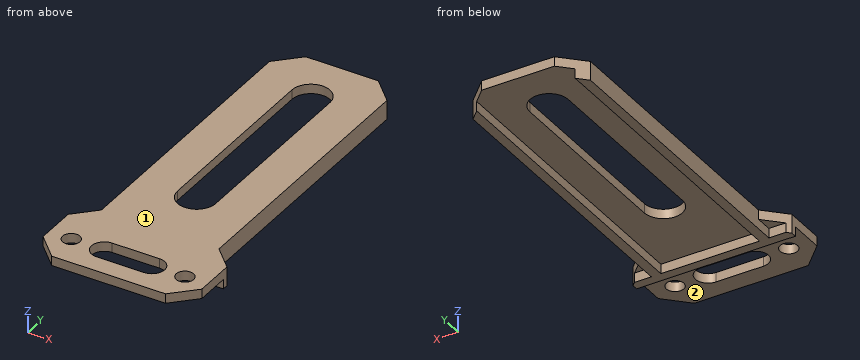
```python
from build123d import *

# Parameters (mm, degrees)
SKETCH1_R           = 2.75
BOSS_EXTRUDE1_DEPTH = 3
BOSS_EXTRUDE2_DEPTH = 3


with BuildPart() as part:
    # Sketch1 → Boss-Extrude1 (new body)
    with BuildSketch(Plane.XY):
        Polygon((7.071067812, 0), (42.928932188, 0), (50, 7.071067812), (50, 20), (43.5, 26.5), (43.5, 112.928932188), (36.428932188, 120), (13.571067812, 120), (6.5, 112.928932188), (6.5, 26.5), (0, 20), (0, 7.071067812), align=None)
        with Locations((7.1, 10)):
            Circle(SKETCH1_R, mode=Mode.SUBTRACT)
        with Locations(Location((42.9, 10, 0), (0, 0, 180))):
            Circle(SKETCH1_R, mode=Mode.SUBTRACT)
        with BuildLine():
            Line((19, 45.27), (19, 104))
            ThreePointArc((19, 104), (25, 110), (31, 104))
            Line((31, 104), (31, 45.27))
            ThreePointArc((31, 45.27), (25, 39.27), (19, 45.27))
        make_face(mode=Mode.SUBTRACT)
        with BuildLine():
            Line((17.5, 14), (32.5, 14))
            ThreePointArc((32.5, 14), (36.5, 10), (32.5, 6))
            Line((32.5, 6), (17.5, 6))
            ThreePointArc((17.5, 6), (13.5, 10), (17.5, 14))
        make_face(mode=Mode.SUBTRACT)
    extrude(amount=BOSS_EXTRUDE1_DEPTH)

    # Sketch2 → Boss-Extrude2 (add)
    with BuildSketch(Plane(origin=(0, 0, 0), x_dir=(-1, 0, 0), z_dir=(0, 0, -1))):
        Polygon((-50, 18.19), (0, 18.19), (0, 20), (-1.19, 21.19), (-6.5, 21.19), (-6.5, 112.928932188), (-9.5, 115.928932188), (-9.5, 21.19), (-40.5, 21.19), (-40.5, 115.928932188), (-43.5, 112.928932188), (-43.5, 21.19), (-48.81, 21.19), (-50, 20), align=None)
    extrude(amount=BOSS_EXTRUDE2_DEPTH)


solid = part.part
```
Input: part model. Units: mm. Frame: model coordinates. Face numbers are marked on the shaded views. Give positions to 0.01 mm unless a question says otherwise; leave off trailing zeros. Order: outer loops, then holes, each group sorted by start corner. A loop starts at its lowest first (then second) coordinate and runs counter-clockwise, first axis right, second up.
1. Section B-B on z = 1.15. Return the cut outline in (x, y), and give its area (3 significant figures).
Derived:
outline: (0, 7.07) - (7.07, 0) - (42.93, 0) - (50, 7.07) - (50, 20) - (43.5, 26.5) - (43.5, 112.93) - (36.43, 120) - (13.57, 120) - (6.5, 112.93) - (6.5, 26.5) - (0, 20) - close; hole circle Ø5.5 at (7.1, 10); hole (17.5, 6) - (32.5, 6) arc R4 ccw to (32.5, 14) - (17.5, 14) arc R4 ccw to start; hole (19, 45.27) arc R6 ccw to (31, 45.27) - (31, 104) arc R6 ccw to (19, 104) - close; hole circle Ø5.5 at (42.9, 10)
area: 3,610 mm2
2. Pin query (flat end, axial travel): pin 1 (5.5 mm diameter, centred on x = 22, y = 5, fed in from -Z); pin 2 (0.9 mm diameter, centred on y = 81, z = 1.5, fed in from -X); pin 3 (4.5 mm diameter, centred on x = 7.1, y = 10, fed in from +Z); pin 4 (2.5 mm diameter, centred on x = 46.5, z = -2, fed in from +Y). Return the tip coordinate at first contact, or that it passes through.
Derived:
pin 1: stops at z = 0
pin 2: stops at x = 6.5
pin 3: passes through
pin 4: stops at y = 21.19
3. Material intervals for L1, parallel to Y at x = 25, z = 1.6; L2, parallel to X at y = 58.5, z = 2.75; L3, parallel to X at y = 11.5, z = 1.15, sorted ascending.
Derived:
L1: y = 0 to 6, 14 to 39.27, 110 to 120
L2: x = 6.5 to 19, 31 to 43.5
L3: x = 0 to 4.8, 9.4 to 13.79, 36.21 to 40.6, 45.2 to 50
4. Section A-A on x = 25. Return the cut outline in (y, z), and give its area (3 significant figures).
Derived:
outline: (0, 0) - (6, 0) - (6, 3) - (0, 3) - close; (14, 0) - (18.19, 0) - (18.19, -3) - (21.19, -3) - (21.19, 0) - (39.27, 0) - (39.27, 3) - (14, 3) - close; (110, 0) - (120, 0) - (120, 3) - (110, 3) - close
area: 133 mm2
5. Section D-D on y = 85.5. Return the cut outline in (x, z).
Derived:
outline: (6.5, -3) - (9.5, -3) - (9.5, 0) - (19, 0) - (19, 3) - (6.5, 3) - close; (31, 0) - (40.5, 0) - (40.5, -3) - (43.5, -3) - (43.5, 3) - (31, 3) - close
6. Mould query, pull axis Z, two halves, no side actions, for the marked faces 1 and 2. Classes: released by +Z, released by -Z, zero draft, split by the parting line, or undercut.
Derived:
face 1: released by +Z
face 2: released by -Z
7. Section C-C on y = 10. Return the cut outline in (x, z), and give its area (3 significant figures).
Derived:
outline: (0, 0) - (4.35, 0) - (4.35, 3) - (0, 3) - close; (9.85, 0) - (13.5, 0) - (13.5, 3) - (9.85, 3) - close; (36.5, 0) - (40.15, 0) - (40.15, 3) - (36.5, 3) - close; (45.65, 0) - (50, 0) - (50, 3) - (45.65, 3) - close
area: 48.0 mm2
